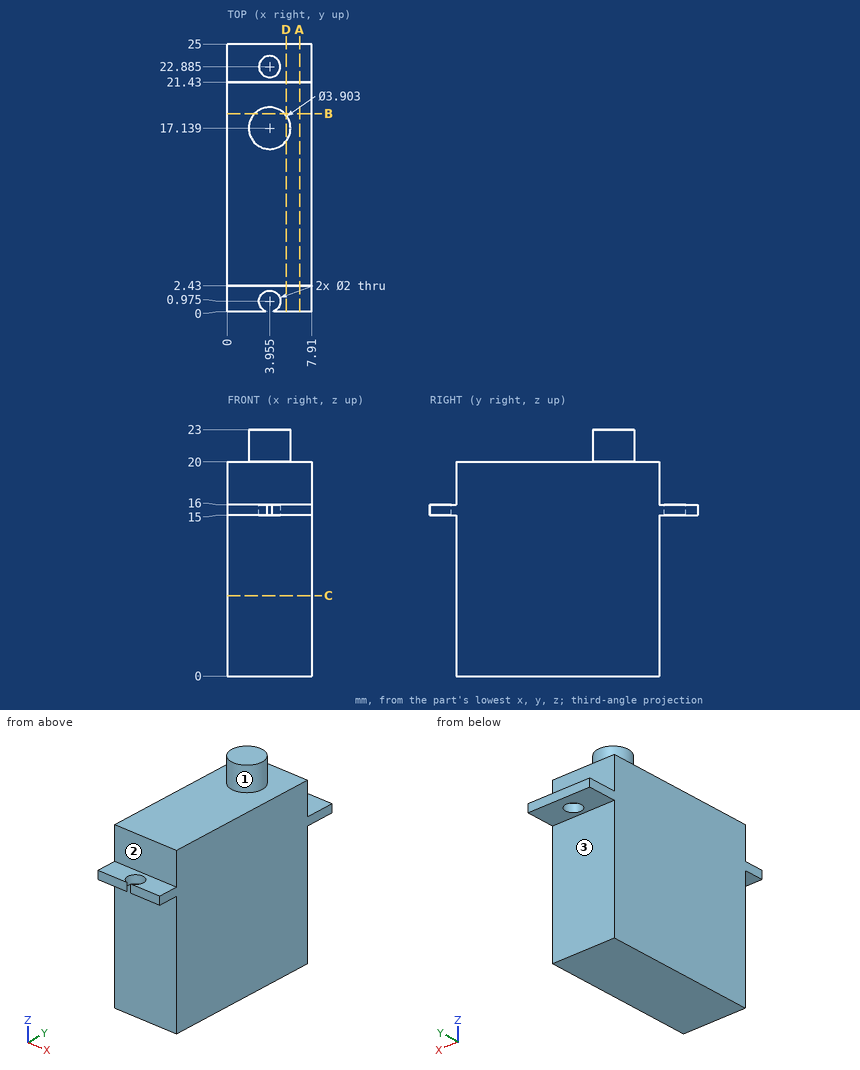
For this review, use the dimensioned drawing (mm, ordinates from the lowest corner) and the shaded views. A direction names the side the tool comes from. Round coordinates to 2 decimals unless told otherwise and drop trailing zeros. Write each loop counter-clockwise with the first axis right and the second up, starting at its lowest first coordinate (ties: lowest second). Pieces come first, ordered by that corner, then holes. Notation, with made-up numbers: (-1.75, 84) - (27.25, 84) arc R23 cw to (27.25, 109) - close; hole circle Ø1 at (73.5, 74). An arc over 180 degrees is marked (long way). Answer as CSV lines item,"result". Start each with the question number.
(1) We need section B-B on y = 18.5. State the section outline as (x, z) points.
(2) We need section D-D on x = 5.5. State the section outline as (y, z) points, plus the area to 3 significant figures.
(3) For the marked faces 1, 2 and 3, list the 3-axis set-ups (+Z, -Z, +X, -X, +Y, -Y) from which the entire face can be reached by the end or side of a thin tool; tool diameter is ignored.
(4) We need section A-A on x = 6.75. State the section outline as (y, z) points.
(5) We need section C-C on z = 7.5. State the section outline as (x, y) points.
(6) For pin 1 Ø1.2 at (x, z) = (3.5, 18.5) entering from -Y; pin 2 Ø4 at (x, z) = (1, 8) entering from +Y; pin 3 Ø1.1 at (x, y) = (4.5, 22.5) entering from -Z; pin 4 Ø1.5 at (x, y) = (4.5, 4) entering from -Z, all flat-tipped, find the tip position at first contact; note any pin that passes through.
(7) To check wall thickness, follow line 1 (Z direction, x = 4.5, y = 10.5); line 2 (Y direction, x = 7, z = 16.25); line 3 (Z direction, x = 3.25, y = 24.25). State the ranges of each line that lie inside material, in increasing order.
Worked answers:
1,outline,"(0, 0) - (7.91, 0) - (7.91, 20) - (5.35, 20) - (5.35, 23) - (2.56, 23) - (2.56, 20) - (0, 20) - close"
2,outline,"(0, 15) - (2.43, 15) - (2.43, 0) - (21.43, 0) - (21.43, 15) - (25, 15) - (25, 16) - (21.43, 16) - (21.43, 20) - (18.33, 20) - (18.33, 23) - (15.95, 23) - (15.95, 20) - (2.43, 20) - (2.43, 16) - (0, 16) - close"
2,area,"393 mm²"
3,face 1,"+Z"
3,face 2,"+Z, +X, -X, -Y"
3,face 3,"-Z, +X, -X, +Y"
4,outline,"(0, 15) - (2.43, 15) - (2.43, 0) - (21.43, 0) - (21.43, 15) - (25, 15) - (25, 16) - (21.43, 16) - (21.43, 20) - (2.43, 20) - (2.43, 16) - (0, 16) - close"
5,outline,"(0, 2.43) - (7.91, 2.43) - (7.91, 21.43) - (0, 21.43) - close"
6,pin 1,"y = 2.43"
6,pin 2,"y = 21.43"
6,pin 3,"z = 15"
6,pin 4,"z = 0"
7,line 1,"0 to 20"
7,line 2,"2.43 to 21.43"
7,line 3,"15 to 16"
